Model file for the job. Use its own axes, mm. Give positions to 0.01 mm unless a question says otherwise; leave off trailing zeros. Write each loop counter-clockwise with the first axis right and the second up, starting at its lowest first coordinate (ties: lowest second). Pieces come first, ordered by that corner, then holes.
Autodesk Inventor part; units mm, degrees
ref_plane "YZ Plane" through (0, 0, 0) normal (1, 0, 0) x (0, 1, 0)
ref_plane "XZ Plane" through (0, 0, 0) normal (0, 1, 0) x (-1, 0, 0)
ref_plane "XY Plane" through (0, 0, 0) normal (0, 0, 1) x (1, 0, 0)
sketch "Sketch2" plane through (0, 0, 0) normal (0, 0, 1) x (1, 0, 0)
  line L0 (7.62, 67.0577) -> (50.8, 67.0577)
  line L1 (50.8, 67.0577) -> (50.8, 16.2577)
  line L2 (50.8, 16.2577) -> (7.62, 16.2577)
  line L3 (7.62, 16.2577) -> (7.62, 67.0577)
  point P0 (0, 0)
  dimension "d45" = 43.18
  dimension "d46" = 50.8
extrude "Extrusion1" add sketch "Sketch2" along normal blind 2.54
sketch "Sketch3" plane through (0, 0, 0) normal (0, 0, -1) x (-1, 0, 0)
  circle A0 centre (-43.18, 59.4377) radius 4.0005
  line L0 (-50.8, 16.2577) -> (-50.8, 67.0577)
  line L1 (-50.8, 67.0577) -> (-7.62, 67.0577)
  circle A1 centre (-43.18, 59.4377) radius 5.2705
  line L2 (-7.62, 67.0577) -> (-7.62, 16.2577)
  line L3 (-7.62, 16.2577) -> (-50.8, 16.2577)
  circle A2 centre (-43.18, 46.7377) radius 5.2705
  circle A3 centre (-30.48, 59.4377) radius 5.2705
  circle A4 centre (-30.48, 46.7377) radius 5.2705
  circle A5 centre (-17.78, 59.4377) radius 5.2705
  circle A6 centre (-17.78, 46.7377) radius 5.2705
  line L4 (-45.1739, 39.1092) -> (-41.1861, 39.1092)
  line L5 (-41.1861, 39.1092) -> (-41.1861, 36.0358)
  line L6 (-41.1861, 36.0358) -> (-45.1739, 36.0358)
  line L7 (-45.1739, 36.0358) -> (-45.1739, 39.1092)
  line L8 (-45.1739, 39.1092) -> (-41.1861, 36.0358) construction
  line L9 (-41.1861, 39.1092) -> (-45.1739, 36.0358) construction
  line L10 (-45.9813, 35.4135) -> (-40.3787, 35.4135)
  line L11 (-40.3787, 35.4135) -> (-40.3787, 39.7315)
  line L12 (-40.3787, 39.7315) -> (-45.9813, 39.7315)
  line L13 (-45.9813, 39.7315) -> (-45.9813, 35.4135)
  line L14 (-45.9813, 35.4135) -> (-40.3787, 39.7315) construction
  line L15 (-40.3787, 35.4135) -> (-45.9813, 39.7315) construction
  circle A7 centre (-30.48, 59.4377) radius 4.1255
  circle A8 centre (-17.78, 59.4377) radius 4.2505
  circle A9 centre (-43.18, 46.7377) radius 4.3755
  circle A10 centre (-30.48, 46.7377) radius 4.5005
  circle A11 centre (-17.78, 46.7377) radius 4.6255
  line L16 (-32.7587, 39.7315) -> (-38.3613, 39.7315)
  line L17 (-38.3613, 39.7315) -> (-38.3613, 35.4135)
  line L18 (-38.3613, 35.4135) -> (-32.7587, 35.4135)
  line L19 (-32.7587, 35.4135) -> (-32.7587, 39.7315)
  line L20 (-25.1387, 39.7315) -> (-30.7413, 39.7315)
  line L21 (-30.7413, 39.7315) -> (-30.7413, 35.4135)
  line L22 (-30.7413, 35.4135) -> (-25.1387, 35.4135)
  line L23 (-25.1387, 35.4135) -> (-25.1387, 39.7315)
  line L24 (-17.5187, 39.7315) -> (-23.1213, 39.7315)
  line L25 (-23.1213, 39.7315) -> (-23.1213, 35.4135)
  line L26 (-23.1213, 35.4135) -> (-17.5187, 35.4135)
  line L27 (-17.5187, 35.4135) -> (-17.5187, 39.7315)
  line L28 (-9.8987, 39.7315) -> (-15.5013, 39.7315)
  line L29 (-15.5013, 39.7315) -> (-15.5013, 35.4135)
  line L30 (-15.5013, 35.4135) -> (-9.8987, 35.4135)
  line L31 (-9.8987, 35.4135) -> (-9.8987, 39.7315)
  line L32 (-37.6789, 35.9108) -> (-33.4411, 35.9108)
  line L33 (-33.4411, 35.9108) -> (-33.4411, 39.2342)
  line L34 (-33.4411, 39.2342) -> (-37.6789, 39.2342)
  line L35 (-37.6789, 39.2342) -> (-37.6789, 35.9108)
  line L36 (-37.6789, 35.9108) -> (-33.4411, 39.2342) construction
  line L37 (-33.4411, 35.9108) -> (-37.6789, 39.2342) construction
  line L38 (-30.1839, 35.7858) -> (-25.6961, 35.7858)
  line L39 (-25.6961, 35.7858) -> (-25.6961, 39.3592)
  line L40 (-25.6961, 39.3592) -> (-30.1839, 39.3592)
  line L41 (-30.1839, 39.3592) -> (-30.1839, 35.7858)
  line L42 (-30.1839, 35.7858) -> (-25.6961, 39.3592) construction
  line L43 (-25.6961, 35.7858) -> (-30.1839, 39.3592) construction
  line L44 (-22.6889, 35.6608) -> (-17.9511, 35.6608)
  line L45 (-17.9511, 35.6608) -> (-17.9511, 39.4842)
  line L46 (-17.9511, 39.4842) -> (-22.6889, 39.4842)
  line L47 (-22.6889, 39.4842) -> (-22.6889, 35.6608)
  line L48 (-22.6889, 35.6608) -> (-17.9511, 39.4842) construction
  line L49 (-17.9511, 35.6608) -> (-22.6889, 39.4842) construction
  line L50 (-45.1739, 35.3552) -> (-41.1861, 35.3552)
  line L51 (-41.1861, 35.3552) -> (-41.1861, 36.7164)
  line L52 (-41.1861, 36.7164) -> (-45.1739, 36.7164)
  line L53 (-45.1739, 36.7164) -> (-45.1739, 35.3552)
  line L54 (-45.1739, 35.3552) -> (-41.1861, 36.7164) construction
  line L55 (-41.1861, 35.3552) -> (-45.1739, 36.7164) construction
  point P0 (0, 0)
  point P1 (-43.18, 37.5725)
  point P2 (-43.18, 37.5725)
  point P3 (-35.56, 37.5725)
  point P4 (-27.94, 37.5725)
  point P5 (-20.32, 37.5725)
  point P6 (-12.7, 37.5725)
  point P7 (-43.18, 36.0358)
  dimension "d49" = 7.62
  dimension "d50" = 7.62
  dimension "d51" = 1.27
  dimension "d56" = 12.7
  dimension "d59" = 12.7
  dimension "d64" = 3.9878
  dimension "d65" = 3.0734
  dimension "d66" = 9.1652
  dimension "d67" = 2.159
  dimension "d77" = 8.001
  dimension "d78" = 8.251
  dimension "d80" = 8.501
  dimension "d81" = 8.751
  dimension "d82" = 9.001
  dimension "d83" = 9.251
  dimension "d90" = 7.62
  dimension "d95" = 4.2378
  dimension "d96" = 4.4878
  dimension "d97" = 4.7378
  dimension "d98" = 3.3234
  dimension "d99" = 3.5734
sketch "Sketch4" plane through (0, 0, 0) normal (0, 0, -1) x (-1, 0, 0)
  line L0 (-50.8, 67.0577) -> (-7.62, 67.0577)
  line L1 (-50.8, 16.2577) -> (-50.8, 67.0577)
  line L2 (-50.8, 67.0577) -> (-48.5295, 67.0577)
  line L3 (-48.5295, 67.0577) -> (-48.5295, 65.0024)
  line L4 (-48.5295, 65.0024) -> (-50.8, 65.0024)
  line L5 (-50.8, 65.0024) -> (-50.8, 67.0577)
  point P0 (0, 0)
extrude "Extrusion3" cut sketch "Sketch4" against normal blind 2.54
sketch "Sketch5" plane through (0, 0, 0) normal (0, 0, -1) x (-1, 0, 0)
  line L0 (-45.1739, 39.1092) -> (-41.1861, 39.1092)
  line L1 (-41.1861, 39.1092) -> (-41.1861, 36.0358)
  line L2 (-41.1861, 36.0358) -> (-45.1739, 36.0358)
  line L3 (-45.1739, 36.0358) -> (-45.1739, 39.1092)
  line L4 (-45.1739, 39.1092) -> (-41.1861, 36.0358) construction
  line L5 (-41.1861, 39.1092) -> (-45.1739, 36.0358) construction
  line L6 (-45.9813, 35.4135) -> (-40.3787, 35.4135)
  line L7 (-40.3787, 35.4135) -> (-40.3787, 39.7315)
  line L8 (-40.3787, 39.7315) -> (-45.9813, 39.7315)
  line L9 (-45.9813, 39.7315) -> (-45.9813, 35.4135)
  line L10 (-45.9813, 35.4135) -> (-40.3787, 39.7315) construction
  line L11 (-40.3787, 35.4135) -> (-45.9813, 39.7315) construction
  line L12 (-32.7587, 39.7315) -> (-38.3613, 39.7315)
  line L13 (-38.3613, 39.7315) -> (-38.3613, 35.4135)
  line L14 (-38.3613, 35.4135) -> (-32.7587, 35.4135)
  line L15 (-32.7587, 35.4135) -> (-32.7587, 39.7315)
  line L16 (-25.1387, 39.7315) -> (-30.7413, 39.7315)
  line L17 (-30.7413, 39.7315) -> (-30.7413, 35.4135)
  line L18 (-30.7413, 35.4135) -> (-25.1387, 35.4135)
  line L19 (-25.1387, 35.4135) -> (-25.1387, 39.7315)
  line L20 (-17.5187, 39.7315) -> (-23.1213, 39.7315)
  line L21 (-23.1213, 39.7315) -> (-23.1213, 35.4135)
  line L22 (-23.1213, 35.4135) -> (-17.5187, 35.4135)
  line L23 (-17.5187, 35.4135) -> (-17.5187, 39.7315)
  line L24 (-9.8987, 39.7315) -> (-15.5013, 39.7315)
  line L25 (-15.5013, 39.7315) -> (-15.5013, 35.4135)
  line L26 (-15.5013, 35.4135) -> (-9.8987, 35.4135)
  line L27 (-37.6789, 35.9108) -> (-33.4411, 35.9108)
  line L28 (-33.4411, 35.9108) -> (-33.4411, 39.2342)
  line L29 (-33.4411, 39.2342) -> (-37.6789, 39.2342)
  line L30 (-37.6789, 39.2342) -> (-37.6789, 35.9108)
  line L31 (-37.6789, 35.9108) -> (-33.4411, 39.2342) construction
  line L32 (-33.4411, 35.9108) -> (-37.6789, 39.2342) construction
  line L33 (-30.1839, 35.7858) -> (-25.6961, 35.7858)
  line L34 (-25.6961, 35.7858) -> (-25.6961, 39.3592)
  line L35 (-25.6961, 39.3592) -> (-30.1839, 39.3592)
  line L36 (-30.1839, 39.3592) -> (-30.1839, 35.7858)
  line L37 (-30.1839, 35.7858) -> (-25.6961, 39.3592) construction
  line L38 (-25.6961, 35.7858) -> (-30.1839, 39.3592) construction
  line L39 (-22.6889, 35.6608) -> (-17.9511, 35.6608)
  line L40 (-17.9511, 35.6608) -> (-17.9511, 39.4842)
  line L41 (-17.9511, 39.4842) -> (-22.6889, 39.4842)
  line L42 (-22.6889, 39.4842) -> (-22.6889, 35.6608)
  line L43 (-22.6889, 35.6608) -> (-17.9511, 39.4842) construction
  line L44 (-17.9511, 35.6608) -> (-22.6889, 39.4842) construction
  line L45 (-45.1516, 35.2931) -> (-41.1861, 36.7869) construction
  line L46 (-41.1861, 35.3552) -> (-45.1739, 36.7164) construction
  line L47 (-44.9867, 35.3552) -> (-41.3733, 35.3552)
  line L48 (-41.3733, 35.3552) -> (-41.3733, 36.7164)
  line L49 (-41.3733, 36.7164) -> (-44.9867, 36.7164)
  line L50 (-44.9867, 36.7164) -> (-44.9867, 35.3552)
  line L51 (-44.9867, 35.3552) -> (-41.3733, 36.7164) construction
  line L52 (-41.3733, 35.3552) -> (-44.9867, 36.7164) construction
  line L53 (-37.5427, 35.3747) -> (-33.5773, 35.3747)
  line L54 (-33.5773, 35.3747) -> (-33.5773, 36.447)
  line L55 (-33.5773, 36.447) -> (-37.5427, 36.447)
  line L56 (-37.5427, 36.447) -> (-37.5427, 35.3747)
  line L57 (-37.5427, 35.3747) -> (-33.5773, 36.447) construction
  line L58 (-33.5773, 35.3747) -> (-37.5427, 36.447) construction
  line L59 (-30.0124, 35.3468) -> (-25.8676, 35.3468)
  line L60 (-25.8676, 35.3468) -> (-25.8676, 36.2248)
  line L61 (-25.8676, 36.2248) -> (-30.0124, 36.2248)
  line L62 (-30.0124, 36.2248) -> (-30.0124, 35.3468)
  line L63 (-30.0124, 35.3468) -> (-25.8676, 36.2248) construction
  line L64 (-25.8676, 35.3468) -> (-30.0124, 36.2248) construction
  line L65 (-22.4558, 35.2013) -> (-18.1842, 35.2013)
  line L66 (-18.1842, 35.2013) -> (-18.1842, 36.1203)
  line L67 (-18.1842, 36.1203) -> (-22.4558, 36.1203)
  line L68 (-22.4558, 36.1203) -> (-22.4558, 35.2013)
  line L69 (-22.4558, 35.2013) -> (-18.1842, 36.1203) construction
  line L70 (-18.1842, 35.2013) -> (-22.4558, 36.1203) construction
  line L71 (-45.9813, 32.6353) -> (-41.9935, 32.6353)
  line L72 (-41.9935, 32.6353) -> (-41.9935, 29.5619)
  line L73 (-41.9935, 29.5619) -> (-45.9813, 29.5619)
  line L74 (-45.9813, 29.5619) -> (-45.9813, 32.6353)
  point P0 (0, 0)
  point P1 (-43.18, 37.5725)
  point P2 (-43.18, 37.5725)
  point P3 (-35.56, 37.5725)
  point P4 (-27.94, 37.5725)
  point P5 (-20.32, 37.5725)
  point P6 (-12.7, 37.5725)
  point P7 (-43.18, 36.0358)
  point P8 (-35.56, 35.9108)
  point P9 (-27.94, 35.7858)
  point P10 (-20.32, 35.6608)
  point P11 (-22.4558, 35.4135)
  point P12 (-22.4558, 35.6608)
  point P13 (-18.1842, 35.6608)
  point P14 (-18.1842, 35.4135)
  point P15 (-30.0124, 35.4135)
  point P16 (-30.0124, 35.7858)
  point P17 (-25.8676, 35.7858)
  point P18 (-25.8676, 35.4135)
  point P19 (-37.5427, 35.4135)
  point P20 (-37.5427, 35.9108)
  point P21 (-33.5773, 35.9108)
  point P22 (-33.5773, 35.4135)
  point P23 (-44.9867, 35.4135)
  point P24 (-44.9867, 36.0358)
  point P25 (-41.3733, 36.0358)
  point P26 (-41.3733, 35.4135)
  dimension "d102" = 3.0734
  dimension "d103" = 2.159
  dimension "d104" = 7.62
  dimension "d106" = 4.4878
  dimension "d107" = 4.7378
  dimension "d108" = 3.3234
  dimension "d109" = 3.5734
  dimension "d114" = 4.2378
  dimension "d115" = 3.0734
  dimension "d116" = 3.9878
extrude "Extrusion5" add sketch "Sketch5" along normal blind 2.54 contours L3 L2 L50 L6 L9 L8 L7 L48 L1 L0 | L15 L14 L54 L27 L28 L29 L30 L56 L13 L12 | L19 L18 L60 L33 L34 L35 L36 L62 L17 L16 | L23 L22 L66 L39 L40 L41 L42 L68 L21 L20
sketch "Sketch6" plane through (0, 0, 0) normal (0, 0, -1) x (-1, 0, 0)
  line L0 (-52.3953, 34.0161) -> (-4.7261, 34.0161)
  line L1 (-4.7261, 34.0161) -> (-4.7261, 12.2528)
  line L2 (-4.7261, 12.2528) -> (-52.3953, 12.2528)
  line L3 (-52.3953, 12.2528) -> (-52.3953, 34.0161)
  point P0 (0, 0)
extrude "Extrusion6" cut sketch "Sketch6" against normal blind 2.54
properties part number "magnet_hall_testing"
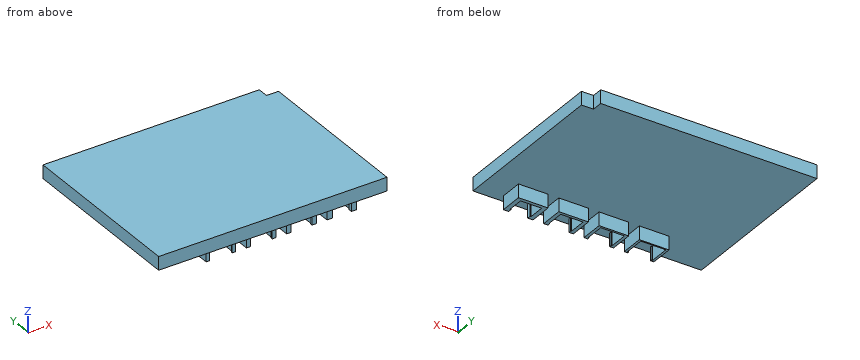
1. Slice it at A-A, the plane x = 37. Write the cut outline in (y, z), and give its area (3 significant figures).
Calculated:
outline: (34.02, 0) - (39.23, 0) - (39.23, -2.54) - (39.73, -2.54) - (39.73, 0) - (67.06, 0) - (67.06, 2.54) - (34.02, 2.54) - close
area: 85.2 mm2
2. Slice it at C-C, the plane x = 44.5. Write the cut outline in (y, z).
Calculated:
outline: (34.02, 0) - (39.11, 0) - (39.11, -2.54) - (39.73, -2.54) - (39.73, 0) - (67.06, 0) - (67.06, 2.54) - (34.02, 2.54) - close
3. Pin check, flat tips, straight feed: P1, Ø1, axis at y = 66.5, z = 1, coming from the +X side; P2, Ø0.8, axis at y = 37, z = -1, coming from the -X side; P3, Ø0.8, axis at x = 40.5, z = -1, coming from the -Y side. Stop position of each tip, or through.
Calculated:
P1: stops at x = 48.53
P2: stops at x = 17.52
P3: stops at y = 35.41
4. Slice it at D-D, the plane y = 43. Write the cut outline in (x, z), and give its area (3 significant figures).
Calculated:
outline: (7.62, 0) - (50.8, 0) - (50.8, 2.54) - (7.62, 2.54) - close
area: 110 mm2
5. Probe probe 1 along Z at (x, y) = (25, 59.5); probe 2 along X at (y, z) = (66, 2.35); probe 3 along Y at (x, z) = (43, -0.85). List the from-to ranges inside material, lowest first.
Calculated:
probe 1: z = 0 to 2.54
probe 2: x = 7.62 to 48.53
probe 3: y = 39.11 to 39.73
6. Slice it at B-B, the plane z = -0.45. State how many separate pieces and enclosed holes the cut face has, and give its area (3 significant figures).
Calculated:
separate pieces: 4
enclosed holes: 0
area: 29.5 mm2
